Autodesk Inventor part; units mm, degrees
ref_plane "YZ Plane" through (0, 0, 0) normal (1, 0, 0) x (0, 1, 0)
ref_plane "XZ Plane" through (0, 0, 0) normal (0, 1, 0) x (-1, 0, 0)
ref_plane "XY Plane" through (0, 0, 0) normal (0, 0, 1) x (1, 0, 0)
sketch "スケッチ1" plane through (0, 0, 0) normal (0, 0, 1) x (1, 0, 0)
  line L0 (-20, 7) -> (20, 7)
  line L1 (20, 7) -> (20, -7)
  line L2 (20, -7) -> (-20, -7)
  line L3 (-20, -7) -> (-20, 7)
  line L4 (-28, 0) -> (28, 0) construction
  line L5 (0, -9.8) -> (0, 9.8) construction
  point P0 (0, 0)
  dimension "d0" = 40
  dimension "d1" = 14
  dimension "d2" = 20
  dimension "d3" = 7
extrude "押し出し1" add sketch "スケッチ1" along normal blind 2
sketch "スケッチ2" plane through (0, 0, 2) normal (0, 0, 1) x (1, 0, 0)
  line L0 (-20, -7) -> (20, -7)
  line L1 (-20, 7) -> (-18, 7)
  line L2 (-18, 7) -> (-18, -7)
  line L3 (-18, -7) -> (-20, -7)
  line L4 (-20, -7) -> (-20, 7)
  point P0 (0, 0)
  dimension "d6" = 2
extrude "押し出し2" add sketch "スケッチ2" along normal blind 23
sketch "スケッチ3" plane through (0, 0, 2) normal (0, 0, 1) x (1, 0, 0)
  line L0 (-18, -7) -> (20, -7)
  line L1 (20, 7) -> (18, 7)
  line L2 (18, 7) -> (18, -7)
  line L3 (18, -7) -> (20, -7)
  line L4 (20, -7) -> (20, 7)
  point P0 (0, 0)
  dimension "d9" = 2
extrude "押し出し3" add sketch "スケッチ3" along normal blind 25
sketch "スケッチ4" plane through (20, -7, 0) normal (1, 0, 0) x (0, 0, -1)
  line L0 (-27, 0) -> (-27, 14)
  circle A0 centre (-20, 7) radius 1.25
  point P0 (0, 7)
  dimension "d12" = 2.5
  dimension "d13" = 7
extrude "押し出し4" cut sketch "スケッチ4" against normal blind 27
sketch "スケッチ5" plane through (20, -7, 0) normal (1, 0, 0) x (0, 0, -1)
  circle A0 centre (-20, 7) radius 1.25
  circle A1 centre (-13.5, 7) radius 0.8
  point P0 (0, 7)
  dimension "d16" = 1.6
  dimension "d17" = 6.5
extrude "押し出し5" cut sketch "スケッチ5" against normal blind 27 contours A1
sketch "スケッチ6" plane through (20, -7, 0) normal (1, 0, 0) x (0, 0, -1)
  circle A0 centre (-20, 7) radius 1.25
  circle A1 centre (-7.5, 7) radius 0.8
  point P0 (0, 7)
  dimension "d20" = 1.6
  dimension "d21" = 12.5
extrude "押し出し6" cut sketch "スケッチ6" against normal blind 27 contours A1
sketch "スケッチ7" plane through (-20, -7, 0) normal (-1, 0, 0) x (0, 0, 1)
  circle A0 centre (20, 7) radius 1.25
  circle A1 centre (20, 7) radius 1.25
  point P0 (0, 7)
  dimension "d24" = 2.5
extrude "押し出し7" cut sketch "スケッチ7" against normal blind 27
sketch "スケッチ8" plane through (0, 0, 2) normal (0, 0, 1) x (1, 0, 0)
  circle A0 centre (-16, 1.5) radius 0.8
  line L0 (-18, -7) -> (18, -7)
  line L1 (0, -9.8) -> (0, 9.8) construction
  line L2 (-20, 7) -> (-20, -7)
  point P0 (0, 0)
  dimension "d27" = 1.6
  dimension "d37" = 8.5
  dimension "d39" = 4
extrude "押し出し8" cut sketch "スケッチ8" against normal blind 27
mirror "ミラー1" about plane through (0, 0, 0) normal (1, 0, 0) of "押し出し8"
chamfer "面取り1" [suppressed]
chamfer "面取り2" distance 3 angle 45 4 edges at (-19, -7, 25) (-19, 7, 25) (19, 7, 27) (19, -7, 27)
sketch "スケッチ9" plane through (0, 0, 0) normal (0, 0, -1) x (-1, 0, 0)
  line L0 (-20, -7) -> (20, -7)
  point P0 (0, 0)
  point P1 (-17, 1)
  dimension "d40" = 8
  dimension "d41" = 17
equation "\"d2\" = 0.5 * d0"
equation "\"d3\" = 0.5 * d1"
properties part number "face"
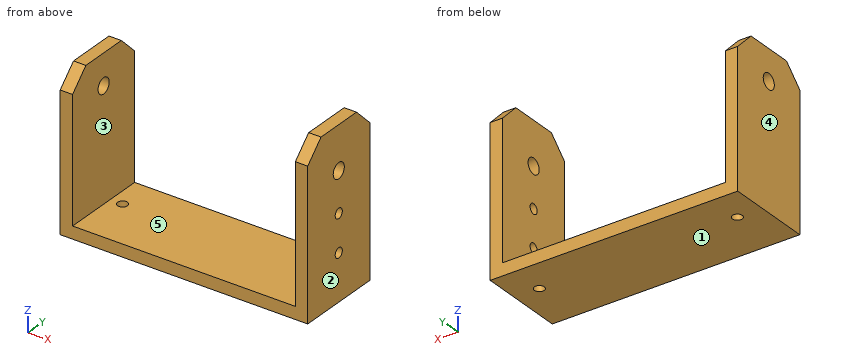
Geometry check sheet. Reference: the model listing, model coordinates, mm. Face numbers are marked on the shaded views. A direction names the side the tool comes from. Coordinates: 2 decimals unless noted, no trailing zeros. Order: outer loops, then holes, each group sorted by start corner. A loop starts at its lowest first (then second) coordinate and runs counter-clockwise, first axis right, second up.
Item 1: Section check C-C (z = 5). Enter the section's corners in (x, y).
Item 2: Depth check by flat-ended pin: pin 1 (2 mm diameter, centred on x = -18.5, y = 1.5, fed in from +Z); pin 2 (6 mm diameter, centred on x = 2.5, y = 2, fed in from +Z). Enter the tip coordinate at first touch or a pass-through.
Item 3: Tool access check on the marked faces 4 and 5. Record the directions out of +Z, -Z, +X, -X, +Y, -Y that give a thin tool (end or side, any length) a straight path to the whole face; none if there is none.
Item 4: Mould release check, pull along X, two halves, no side actions. Record for the marked faces 1, 2 and 3: released by +X, released by -X, zero draft, split by the parting line, or undercut.
Item 5: Section check A-A (y = 0). Enter the section's corners in (x, z).
Item 6: Section check D-D (y = 4.5). Enter the section's corners in (x, z), plus the area to 3 significant figures.
Item 7: Scan lines: line 1 along Y through (x, z) = (18.5, 7.5); line 2 along X through (y, z) = (-4.75, 15.75); line 3 along Z through (x, y) = (-8.5, 3). Record each from-to range of solid material in increasing order.
Item 8: Section check B-B (x = 16). Enter the section's corners in (y, z).
Check sheet entries:
1. outline: (-20, -7) - (-18, -7) - (-18, 7) - (-20, 7) - close; (18, -7) - (20, -7) - (20, 7) - (18, 7) - close
2. pin 1: stops at z = 25
2. pin 2: stops at z = 2
3. face 4: +Z, -Z, -X, +Y, -Y
3. face 5: +Z, +Y, -Y
4. face 1: zero draft
4. face 2: released by +X
4. face 3: undercut
5. outline: (-20, 0) - (20, 0) - (20, 6.7) - (18, 6.7) - (18, 2) - (-18, 2) - (-18, 18.75) - (-20, 18.75) - close; (-20, 21.25) - (-18, 21.25) - (-18, 25) - (-20, 25) - close; (18, 8.3) - (20, 8.3) - (20, 12.7) - (18, 12.7) - close; (18, 14.3) - (20, 14.3) - (20, 18.75) - (18, 18.75) - close; (18, 21.25) - (20, 21.25) - (20, 27) - (18, 27) - close
6. outline: (-20, 0) - (20, 0) - (20, 26.5) - (18, 26.5) - (18, 2) - (-18, 2) - (-18, 24.5) - (-20, 24.5) - close
6. area: 174 mm2
7. line 1: y = -7 to -0.8, 0.8 to 7
7. line 2: x = -20 to -18, 18 to 20
7. line 3: z = 0 to 2
8. outline: (-7, 0) - (0.7, 0) - (0.7, 2) - (-7, 2) - close; (2.3, 0) - (7, 0) - (7, 2) - (2.3, 2) - close
